Part model, mm, in its own coordinate system. A direction names the side the tool comes from. Coordinates: 2 decimals unless noted, no trailing zeros. Loops run counter-clockwise (first coordinate to the right, second up) from the corner with the lowest first, then second, coordinate; pieces in that order, holes last.
Solid Edge part; units mm, degrees
sketch "Sketch1" plane through (0, 0, 0) normal (0, -1, 0) x (1, 0, 0)
  arc A0 (0, 11.5) -> (0, -11.5) centre (0, 0) cw
  line L0 (0, -11.5) -> (-21.5, -11.5)
  line L1 (-21.5, 5) -> (-21.5, -11.5)
  line L2 (-27.1644, 5) -> (-21.5, 5)
  arc A1 (-14.04, 11.5) -> (-27.1644, 5) centre (-14.04, -5) ccw
  line L3 (0, 11.5) -> (-14.04, 11.5)
  dimension "D1" = 21.5
extrude "Protrusion1" add sketch "Sketch1" against normal blind 2
sketch "Sketch2" plane through (-7.8322, 2, 0) normal (0, 1, 0) x (1, 0, 0)
  line L0 (-13.6678, 11.5) -> (7.8322, 11.5)
  arc A0 (7.8322, 11.5) -> (7.8322, -11.5) centre (7.8322, 0) cw
  line L1 (7.8322, -11.5) -> (-6.2078, -11.5)
  arc A1 (-6.2078, -11.5) -> (-19.3322, -5) centre (-6.2078, 5) cw
  line L2 (-19.3322, -5) -> (-17.3881, -5)
  arc A2 (-17.3881, -5) -> (-6.2078, -10) centre (-6.2078, 5) ccw
  line L3 (7.8322, -10) -> (-6.2078, -10)
  arc A3 (7.8322, 10) -> (7.8322, -10) centre (7.8322, 0) cw
  line L4 (-13.6678, 10) -> (7.8322, 10)
  line L5 (-13.6678, 11.5) -> (-13.6678, 10)
  dimension "D1" = 13.6678
extrude "Extrusionsausprägung_2" add sketch "Sketch2" along normal blind 7
chamfer "Fase_1" distance 1 angle 45 4 edges at (-7.02, 9, 11.5) (-21.3629, 9, 9.786) (11.5, 9, 0) (-10.75, 9, -11.5)
sketch "Sketch3" plane through (-7.6102, 2, 0) normal (0, 1, 0) x (1, 0, 0)
  circle A0 centre (7.6102, 0) radius 5
extrude "Cutout1" cut sketch "Sketch3" against normal through all
sketch "Sketch4" plane through (-7.6102, 2, 0) normal (0, 1, 0) x (1, 0, 0)
  line L0 (6.0489, 4.75) -> (-1.9511, 4.75)
  line L1 (-1.9511, 4.75) -> (-1.9511, -4.75)
  line L2 (-1.9511, -4.75) -> (6.0489, -4.75)
  line L3 (6.0489, -4.75) -> (6.0489, 4.75)
  dimension "D1" = 6.0489
  dimension "D2" = 6.0489
extrude "Cutout2" cut sketch "Sketch4" against normal through all
Q1. Drop flat-ended pins along their axis: P1, Ø0.6, axis at x = -23.5, y = 1, coming from the -Z side; P2, Ø2.5, axis at y = 3, z = -4.5, coming from the -X side; P3, Ø1, axis at x = 1, y = 7, coming from the -Z side. Give the stop position or say it passes through.
Q2. Mould opens along X. For faces 1 (the flat face through (-6.9, 8.5, 11)), 2 (the flat face through (-21.5, 1.8, -4.4)), 3 (the flat face through (-12, 2, 0)), 4 (the cylindrical face through (11.497, 3.944, -0.253)) say: released by +X, released by -X, zero draft, split by the parting line, or undercut.
Q3. Tool access for faces 5 (the flat face through (-7, 5, 10)), 6 (the flat face through (-12, 0, 0)), 7 (the flat face through (-6, 1, 4.75)): list every direction of +Z, -Z, +X, -X, +Y, -Y with a clear straight run to the whole face (end or side of a thin tool).
Q4. Probe line 1 (Z direction, x = -7.5, y = 4.75); line 2 (Z direction, x = 0, y = 0.8); line 3 (X direction, y = 6, z = 6.25). List the from-to ranges inside material, lowest first.
Q5. Saw through at A-A (z = 0). List the corners of the cut face in (x, y).
Q6. Saw through at C-C (y = 5.25). List the corners of the cut face in (x, z), plus the area to 3 significant figures.
Checked values:
1. P1: stops at z = 5
1. P2: stops at x = -21.5
1. P3: stops at z = -11.49
2. face 1: zero draft
2. face 2: released by -X
2. face 3: undercut
2. face 4: released by +X
3. face 5: +Y
3. face 6: +Z, -Z, +X, -X, -Y
3. face 7: +Y, -Y
4. line 1: z = -11.5 to -10, 10 to 11.5
4. line 2: z = -11.5 to -5, 5 to 11.5
4. line 3: x = -26.11 to -23.96, 7.81 to 9.65
5. outline: (-21.5, 0) - (-9.56, 0) - (-9.56, 2) - (-21.5, 2) - close; (5, 0) - (11.5, 0) - (11.5, 8) - (10.5, 9) - (10, 9) - (10, 2) - (5, 2) - close
6. outline: (-27.16, 5) - (-25.22, 5) arc R15 cw to (-14.04, 10) - (0, 10) arc R10 cw to (0, -10) - (-21.5, -10) - (-21.5, -11.5) - (0, -11.5) arc R11.5 ccw to (0, 11.5) - (-14.04, 11.5) arc R16.5 ccw to start
6. area: 125 mm2
